from build123d import *

# Parameters (mm, degrees)
ESTRUSIONE_ESTRUSIONE1_DEPTH                         = 3
ESTRUSIONE_ESTRUSIONE1_DEPTH_BACK                    = 12
TAGLIO_ESTRUSIONE1_DEPTH                             = 3
FORO_LAMATO_PER_VITE_M6_A_TESTA_CILINDRI_D           = 6.4
FORO_LAMATO_PER_VITE_M6_A_TESTA_CILINDRI_CBORE_D     = 11
FORO_LAMATO_PER_VITE_M6_A_TESTA_CILINDRI_CBORE_DEPTH = 6.4
FORO_PER_VITE_M6_2_D                                 = 6.6
RIPETIZIONECIRCOLARE1_COUNT                          = 2


with BuildPart() as part:
    # Schizzo1 → Estrusione-Estrusione1 (new body, two sides)
    with BuildSketch(Plane.XY) as estrusione_estrusione1_sk:
        with BuildLine():
            Line((-57.5, -251.4), (57.5, -251.4))
            ThreePointArc((57.5, -251.4), (64.571067812, -248.471067812), (67.5, -241.4))
            Line((67.5, -241.4), (67.5, 162.5))
            ThreePointArc((67.5, 162.5), (64.571067812, 169.571067812), (57.5, 172.5))
            Line((57.5, 172.5), (-57.5, 172.5))
            ThreePointArc((-57.5, 172.5), (-64.571067812, 169.571067812), (-67.5, 162.5))
            Line((-67.5, 162.5), (-67.5, -241.4))
            ThreePointArc((-67.5, -241.4), (-64.571067812, -248.471067812), (-57.5, -251.4))
        make_face()
    extrude(amount=ESTRUSIONE_ESTRUSIONE1_DEPTH)
    extrude(estrusione_estrusione1_sk.sketch, amount=-ESTRUSIONE_ESTRUSIONE1_DEPTH_BACK)

    # Schizzo2 → Taglio-Estrusione1 (cut)
    with BuildSketch(Plane.XY.offset(3)):
        with BuildLine():
            Line((-45, -173.872135955), (-45, -251.4))
            Line((-45, -251.4), (45, -251.4))
            Line((45, -251.4), (45, -173.740515135))
            ThreePointArc((45, -173.740515135), (45.167973297, -172.938219578), (45.643678161, -172.270688251))
            ThreePointArc((45.643678161, -172.270688251), (45.715503432, -166.459321985), (39.909116924, -166.710344828))
            ThreePointArc((39.909116924, -166.710344828), (39.228612943, -167.219435305), (38.398158145, -167.4))
            Line((38.398158145, -167.4), (-38.527864045, -167.4))
            ThreePointArc((-38.527864045, -167.4), (-39.344360626, -167.225741858), (-40.01857603, -166.733333333))
            ThreePointArc((-40.01857603, -166.733333333), (-45.828427125, -166.571572875), (-45.666666667, -172.38142397))
            ThreePointArc((-45.666666667, -172.38142397), (-45.174258142, -173.055639374), (-45, -173.872135955))
        make_face()
    taglio_estrusione1 = extrude(amount=-TAGLIO_ESTRUSIONE1_DEPTH, mode=Mode.SUBTRACT)

    # Foro lamato per Vite M6 a testa cilindri (through all)
    with Locations(Plane(origin=(0, 0, -12), x_dir=(-1, 0, 0), z_dir=(0, 0, -1))):
        with Locations((35.696152423, 97.5), (-22.303847577, 97.5), (-22.303847577, 160.5)):
            foro_lamato_per_vite_m6_a_testa_cilindri = CounterBoreHole(FORO_LAMATO_PER_VITE_M6_A_TESTA_CILINDRI_D / 2, FORO_LAMATO_PER_VITE_M6_A_TESTA_CILINDRI_CBORE_D / 2, FORO_LAMATO_PER_VITE_M6_A_TESTA_CILINDRI_CBORE_DEPTH)

    # Foro per Vite M6-2 (through all)
    with Locations(Plane.XY.offset(3)):
        with Locations((-25, -139.45), (25, 60.55), (25, -139.45), (-25, 60.55), (-25, -39.45), (25, -39.45), (-25, -89.45), (25, -89.45), (-25, 10.55), (25, 10.55), (-95.52986496, -268.984692735)):
            Hole(FORO_PER_VITE_M6_2_D / 2)

    # RipetizioneCircolare1: Taglio-Estrusione1, Foro lamato per Vite M6 a testa cilindri ×2 about axis
    ripetizionecircolare1_axis = Axis((0, -39.45, 0), (0, 0, 1))
    add([taglio_estrusione1.rotate(ripetizionecircolare1_axis, i * 360 / RIPETIZIONECIRCOLARE1_COUNT) for i in range(1, RIPETIZIONECIRCOLARE1_COUNT)], mode=Mode.SUBTRACT)
    add([foro_lamato_per_vite_m6_a_testa_cilindri.rotate(ripetizionecircolare1_axis, i * 360 / RIPETIZIONECIRCOLARE1_COUNT) for i in range(1, RIPETIZIONECIRCOLARE1_COUNT)], mode=Mode.SUBTRACT)


solid = part.part
Check sheet for the modelled part. Datum: model origin and axes. Units: mm. A direction names the side the tool comes from. Round coordinates to 2 decimals unless told otherwise and drop trailing zeros. Loops run counter-clockwise (first coordinate to the right, second up) from the corner with the lowest first, then second, coordinate; pieces in that order, holes last.
1. Gauge pin test, flat ends, axial feed: pin 1 Ø3.5 at (x, z) = (12.5, 1) entering from +Y; pin 2 Ø6 at (x, y) = (-25, -139.45) entering from +Z; pin 3 Ø6.5 at (x, y) = (-22.3, -239.4) entering from +Z; pin 4 Ø3.5 at (x, y) = (-38, 95) entering from -Z. Record the tip position at first contact, or that the pin passes through.
2. Scan lines: probe 1 along X at (y, z) = (-176.4, -8); probe 2 along X at (y, z) = (99.5, -7); probe 3 along Y at (x, z) = (-26.5, -4). Record each from-to range of solid material in increasing order.
3. Sectioned sample at A-A on x = -6. Record the boundary of the cut face in (y, z), and give its area (3 significant figures).
4. Mould release check, pull along X, two halves, no side actions. Record for faces 4 (the cylindrical face through (-23.02, -181.853, -8.845)), 5 (the flat face through (-1, -251.4, -6)), 6 (the cylindrical face through (-64.65, -248.39, -4.39)): released by +X, released by -X, zero draft, split by the parting line, or undercut.
5. Set-up check for faces 1 (the flat face through (-19.9, -174, -5.6)), 2 (the cylindrical face through (-45.78, 87.623, 1.521)), 3 (the flat face through (67.5, -42, -4)): record each of +Z, -Z, +X, -X, +Y, -Y from which the full face is reachable in a straight line by a thin tool's end or side.
Recorded:
1. pin 1: stops at y = 172.5
1. pin 2: passes through
1. pin 3: stops at z = 0
1. pin 4: stops at z = -5.6
2. probe 1: x = -67.5 to -27.8, -16.8 to 30.2, 41.2 to 67.5
2. probe 2: x = -67.5 to -40.82, -30.57 to 17.18, 27.43 to 67.5
2. probe 3: y = -251.4 to -142.39, -136.51 to -92.39, -86.51 to -42.39, -36.51 to 7.61, 13.49 to 57.61, 63.49 to 172.5
3. outline: (-251.4, -12) - (172.5, -12) - (172.5, 0) - (88.5, 0) - (88.5, 3) - (-167.4, 3) - (-167.4, 0) - (-251.4, 0) - close
3. area: 5,850 mm2
4. face 4: undercut
4. face 5: zero draft
4. face 6: released by -X
5. face 1: -Z
5. face 2: +Z
5. face 3: +Z, -Z, +X, +Y, -Y
